from build123d import *

# Parameters (mm, degrees)
SKETCH1_W           = 5
SKETCH1_H           = 4
BOSS_EXTRUDE1_DEPTH = 2
SKETCH2_R           = 0.25
BOSS_EXTRUDE2_DEPTH = 10
FILLET1_SIZE        = 2
FILLET1_SIZE_2      = 1
FILLET2_SIZE        = 1
FILLET2_SIZE_2      = 2


with BuildPart() as part:
    # Sketch1 → Boss-Extrude1 (new body)
    with BuildSketch(Plane(origin=(0, 0, 0), x_dir=(1, 0, 0), z_dir=(0, 1, 0))):
        Rectangle(SKETCH1_W, SKETCH1_H)
    extrude(amount=BOSS_EXTRUDE1_DEPTH)

    # Sketch2 → Boss-Extrude2 (add)
    with BuildSketch(Plane.XZ):
        with Locations(Location((-1.7, 0, 0), (0, 0, 270))):
            Circle(SKETCH2_R)
        with Locations(Location((1.7, 0, 0), (0, 0, 90))):
            Circle(SKETCH2_R)
    extrude(amount=BOSS_EXTRUDE2_DEPTH)

    # Fillet1
    # an asymmetric fillet: 2, 1 mm, written as the material it takes off along each edge
    with BuildSketch(Plane(origin=(-2.5, -5, -2), x_dir=(0, 0, 1), z_dir=(0, 1, 0))) as fillet1_piece_1:
        with BuildLine():
            Bezier((FILLET1_SIZE, 0), (0, 0), (0, FILLET1_SIZE_2), weights=[1, 0.707106781, 1])
            Line((0, FILLET1_SIZE_2), (0, 0))
            Line((0, 0), (FILLET1_SIZE, 0))
        make_face()
    extrude(amount=12, mode=Mode.SUBTRACT)
    with BuildSketch(Plane(origin=(2.5, -5, 2), x_dir=(-1, 0, 0), z_dir=(0, 1, 0))) as fillet1_piece_2:
        with BuildLine():
            Bezier((FILLET1_SIZE_2, 0), (0, 0), (0, -FILLET1_SIZE), weights=[1, 0.707106781, 1])
            Line((0, -FILLET1_SIZE), (0, 0))
            Line((0, 0), (FILLET1_SIZE_2, 0))
        make_face()
    extrude(amount=12, mode=Mode.SUBTRACT)

    # Fillet2
    # an asymmetric fillet: 2, 1 mm, written as the material it takes off along each edge
    with BuildSketch(Plane(origin=(-2.5, -5, 2), x_dir=(1, 0, 0), z_dir=(0, 1, 0)), Plane(origin=(2.5, -5, -2), x_dir=(-1, 0, 0), z_dir=(0, 1, 0))) as fillet2_piece_1:
        with BuildLine():
            Bezier((FILLET2_SIZE, 0), (0, 0), (0, FILLET2_SIZE_2), weights=[1, 0.707106781, 1])
            Line((0, FILLET2_SIZE_2), (0, 0))
            Line((0, 0), (FILLET2_SIZE, 0))
        make_face()
    extrude(amount=12, mode=Mode.SUBTRACT)


solid = part.part
Input: part model. Units: mm. Frame: model coordinates. Coordinates: 2 decimals unless noted, no trailing zeros. Write each loop counter-clockwise with the first axis right and the second up, starting at its lowest first coordinate (ties: lowest second). Pieces come first, ordered by that corner, then holes. Notation, with made-up numbers: M 17.5,-21 L 22.5,-21 A26 cw 22.5,1 Z; hole C 84.25,54 d3. An arc over 180 degrees is marked long. Answer as a JSON object with one key per item and string values. Group by question number.
(1) Contact query for flat-ended pins moving along their axis: P1, Ø2, axis at y = -7.5, z = 0, coming from the -X side; P2, Ø2, axis at x = -0.5, z = -1, coming from the -Y side. Output: stop coordinate, or through.
(2) Section A-A on y = -2.25. Output: boundary loops of the cut face in (x, z), plus the area to 3 significant figures.
(3) Section B-B on x = -0.7. Output: boundary loops of the cut face in (y, z).
(4) Ray query, line 1 along Y through (x, z) = (-1.95, 0.2); line 2 along X through (y, z) = (1.5, 1); line 3 along Z through (x, y) = (1.75, -8). Return the intervals inside material, ascending. Write a range as [from, to].
Result set:
{
 "1": {"P1": "stops at x = -1.95", "P2": "stops at y = 0"},
 "2": {"outline": "C -1.7,0 d0.5; C 1.7,0 d0.5", "area": "0.393 mm2"},
 "3": {"outline": "M 0,-2 L 2,-2 L 2,2 L 0,2 Z"},
 "4": {"line 1": "y = [0, 2]", "line 2": "x = [-2.37, 2.37]", "line 3": "z = [-0.24, 0.24]"}
}
